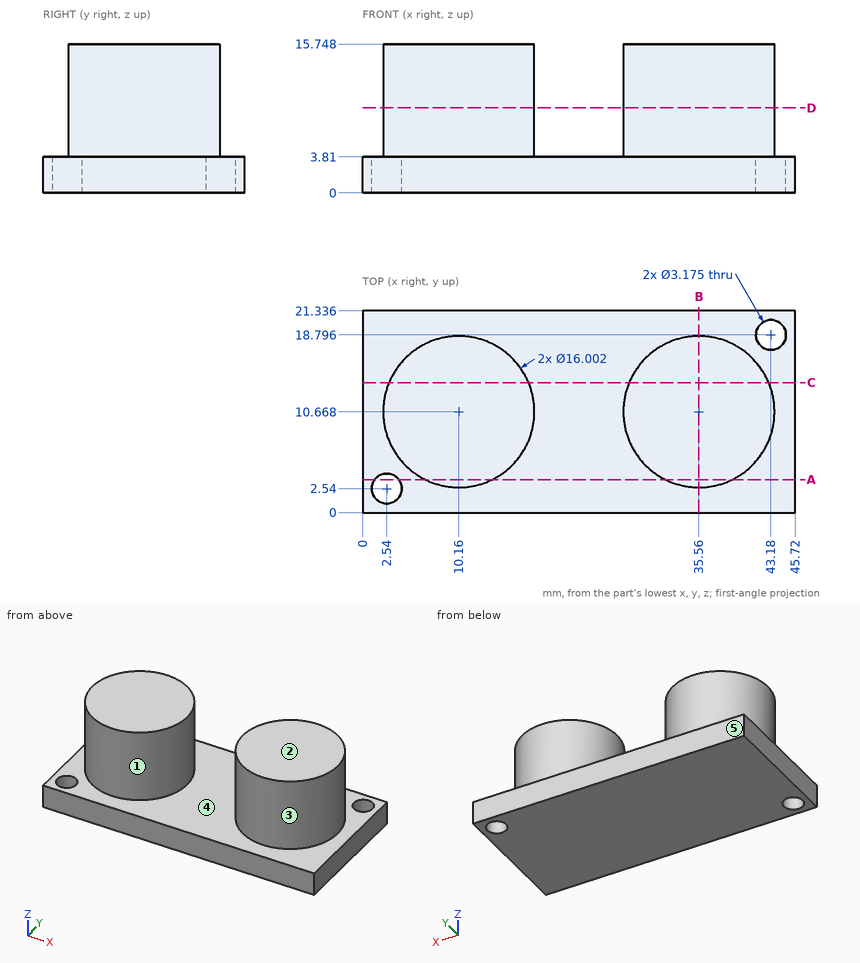
Print and shaded views of the part. All mm, measured from the part's lowest x, y and z. A direction names the side the tool comes from. Coordinates: 2 decimals unless noted, no trailing zeros. Loops run counter-clockwise (first coordinate to the right, second up) from the corner with the lowest first, then second, coordinate; pieces in that order, holes last. Notation, with made-up numbers: (9, 67) - (62, 67) arc R5 cw to (62, 76) - close; hole circle Ø5 at (28.25, -15.5). An arc over 180 degrees is marked (long way). Use one line per item in the form item = value. Start each with the question number.
1) Flat gauge pins, fed straight in: pin 1 (3 mm diameter, centred on x = 40, z = 7, fed in from -Y); pin 2 (6 mm diameter, centred on y = 12, z = 9, fed in from +X); pin 3 (4 mm diameter, centred on x = 12.5, z = 11, fed in from +Y); pin 4 (1.9 mm diameter, centred on x = 2.54, y = 2.54, fed in from -Z). Where does each tip first touch, or does it go through?
2) Band-saw the part on D-D (z = 9). Give the cut face in (x, y).
3) Band-saw the part on A-A (y = 3.5). Give the cut face in (x, z), and give its area (3 significant figures).
4) Tool access for the marked faces 4 and 5: list every direction of +Z, -Z, +X, -X, +Y, -Y with a clear straight run to the whole face (end or side of a thin tool).
5) Drill centre lines: L1, parallel to Y at x = 2.54, z = 1.55; L2, parallel to Y at x = 43.18, z = 1.7; L3, parallel to Z at x = 3, y = 15. Where is each one in solid material? Low to high. Write a range as from..to.
6) Two-plate mould, pull along X, no slides. Class the marked faces 1, 2 and 3: +X half, -X half, draft (parallel to the pull), parting line (faces both ways), or undercut.
7) Band-saw the part on B-B (x = 35.56). Give the cut face in (y, z).
8) Band-saw the part on C-C (y = 13.75). Give the cut face in (x, z).
Check values:
q1.pin_1 = 3.23
q1.pin_2 = 43.56
q1.pin_3 = 18.66
q1.pin_4 = through
q2.outline = circle Ø16 at (10.16, 10.67); circle Ø16 at (35.56, 10.67)
q3.outline = (0, 0) - (1.28, 0) - (1.28, 3.81) - (0, 3.81) - close; (3.8, 0) - (45.72, 0) - (45.72, 3.81) - (39.11, 3.81) - (39.11, 15.75) - (32.01, 15.75) - (32.01, 3.81) - (13.71, 3.81) - (13.71, 15.75) - (6.61, 15.75) - (6.61, 3.81) - (3.8, 3.81) - close
q3.area = 334 mm2
q4.face_4 = +Z
q4.face_5 = +Z, -Z, +X, -X, +Y
q5.L1 = 0..0.95, 4.13..21.34
q5.L2 = 0..17.21, 20.38..21.34
q5.L3 = 0..3.81
q6.face_1 = undercut
q6.face_2 = draft
q6.face_3 = undercut
q7.outline = (0, 0) - (21.34, 0) - (21.34, 3.81) - (18.67, 3.81) - (18.67, 15.75) - (2.67, 15.75) - (2.67, 3.81) - (0, 3.81) - close
q8.outline = (0, 0) - (45.72, 0) - (45.72, 3.81) - (42.94, 3.81) - (42.94, 15.75) - (28.18, 15.75) - (28.18, 3.81) - (17.54, 3.81) - (17.54, 15.75) - (2.78, 15.75) - (2.78, 3.81) - (0, 3.81) - close
